Could you check a few things on this model? Use its own coordinates, in mm. A direction names the side the tool comes from. Round coordinates to 2 decimals unless told otherwise and drop trailing zeros. Write each loop counter-clockwise with the first axis right and the second up, starting at its lowest first coordinate (ties: lowest second). Pieces come first, ordered by that corner, then holes. Notation, with made-up numbers: M 85.25,68.5 L 95.25,68.5 A22 ccw 95.25,92.5 Z; hole C -1.5,34 d10. An arc over 180 degrees is marked long. One line per item, written item: value. Start each with the question number.
(1) I'm going to push flat-ended pins straight in: pin 1 Ø8 at (x, y) = (19.5, 9.5) entering from -Z; pin 2 Ø10 at (x, y) = (6.5, -27) entering from +Z; pin 3 Ø0.8 at (y, z) = (13.5, 1.5) entering from -X; pin 4 Ø2 at (x, z) = (-45, 1) entering from -Y. Where does each tip first touch, or does it pass through?
(2) I want a section at A-A on y = -10. Please give me the cut outline in (x, z).
(3) I want a section at D-D on x = -12. Please give me the cut outline in (y, z).
(4) If I drill on L1, parallel to X at y = 29.5, z = 7; L2, parallel to Z at x = -6.5, y = -33.5, over which ranges is the centre line in solid material (lowest first)?
(5) I want a section at C-C on z = 7. Please give me the cut outline in (x, y).
(6) Which directions (+Z, -Z, +X, -X, +Y, -Y) give clear straight access to the entire face, cutting with the end or side of a thin tool? Please do faces 5 (the face through (58, -1, 6)), 6 (the face through (56.25, -1, 6)), 7 (the face through (-53, 10, 1)).
(7) I want a section at B-B on x = -39. Please give me the cut outline in (y, z), and give its area (3 significant figures).
(8) Thinking about a two-plate mould opening in X: for faces 1 (the face through (-57.14, 0.77, 0.9)), 2 (the face through (-41, -26, 1)), 3 (the face through (-41, 48, 1)), 4 (the face through (0.77, -57.14, 0.9)), which applies, released by +X, released by -X, zero draft, split by the parting line, or undercut?
```python
from build123d import *

# Parameters (mm, degrees)
F0_W     = 116
F0_H     = 116
F0_W_2   = 25
F0_H_2   = 74
F1_DEPTH = 10
F2_W     = 112.5
F2_H     = 112.5
F2_W_2   = 25
F2_H_2   = 74
F3_DEPTH = 7.5
F4_R     = 3


with BuildPart() as f1:
    # F0 (on Top) → F1 (new body)
    with BuildSketch(Plane.XY):
        Rectangle(F0_W, F0_H)
        with Locations((-40.5, 11)):
            Rectangle(F0_W_2, F0_H_2, mode=Mode.SUBTRACT)
    extrude(amount=F1_DEPTH)

    # F2 (on face) → F3 (cut)
    with BuildSketch(Plane.XY.offset(10)):
        Rectangle(F2_W, F2_H)
        with Locations((-40.5, 11)):
            Rectangle(F2_W_2, F2_H_2, mode=Mode.SUBTRACT)
    extrude(amount=-F3_DEPTH, mode=Mode.SUBTRACT)

    # F4
    f4_edges = [f1.edges().sort_by_distance(p)[0] for p in [
        (58, 58, 5),
        (58, -58, 5),
        (-58, 58, 5),
        (-58, -58, 5),
        (-58, 0, 0),
        (0, -58, 0),
        (0, 58, 0),
        (58, 0, 0),
    ]]
    fillet(f4_edges, radius=F4_R)


solid = f1.part
```
Found:
1. pin 1: stops at z = 0
1. pin 2: stops at z = 2.5
1. pin 3: stops at x = -57.79
1. pin 4: stops at y = -57.83
2. outline: M -58,3 A3 ccw -55,0 L -53,0 L -53,2.5 L -56.25,2.5 L -56.25,10 L -58,10 Z; M -28,0 L 55,0 A3 ccw 58,3 L 58,10 L 56.25,10 L 56.25,2.5 L -28,2.5 Z
3. outline: M -58,3 A3 ccw -55,0 L 55,0 A3 ccw 58,3 L 58,10 L 56.25,10 L 56.25,2.5 L -56.25,2.5 L -56.25,10 L -58,10 Z
4. L1: x = -58 to -56.25, 56.25 to 58
4. L2: z = 0 to 2.5
5. outline: M -58,-55 A3 ccw -55,-58 L 55,-58 A3 ccw 58,-55 L 58,55 A3 ccw 55,58 L -55,58 A3 ccw -58,55 Z; hole M -56.25,-56.25 L 56.25,-56.25 L 56.25,56.25 L -56.25,56.25 Z
6. face 5: +Z, -Z, +X, +Y, -Y
6. face 6: +Z
6. face 7: +Z, -Z
7. outline: M -58,3 A3 ccw -55,0 L -26,0 L -26,2.5 L -56.25,2.5 L -56.25,10 L -58,10 Z; M 48,0 L 55,0 A3 ccw 58,3 L 58,10 L 56.25,10 L 56.25,2.5 L 48,2.5 Z
7. area: 127 mm²
8. face 1: released by -X
8. face 2: undercut
8. face 3: undercut
8. face 4: zero draft
